```python
from build123d import *

# Parameters (mm, degrees)
F1_DEPTH    = 30
F2_R        = 10
F3_T1_DEPTH = 56.2345635929
F3_T3_DEPTH = 50.7373541457
F3_T5_DEPTH = 44.5080633868
F3_T7_DEPTH = 55
F4_R        = 1


# Not quite as in the source:
# - a fillet or chamfer that OpenCascade refuses, or shapes differently, is made with other operations: its cross-section is extruded or revolved along the edge and cut away or added


with BuildPart() as f1:
    # F0 (on Right) → F1 (new body)
    with BuildSketch(Plane.YZ):
        Polygon((-27.3037352718, 5), (-27.0568225533, 0), (42.9431774467, 0), (42.9431774467, 5), (25.6962647282, 5), (45.6962647282, 40), (40.6962647282, 40), (20.6962647282, 5), (8.8888889937, 5), (2.6962647282, 5), (2.6962647282, 40), (-2.3037352718, 40), (-2.3037352718, 5), align=None)
    extrude(amount=F1_DEPTH)

    # F2
    f2_edges = [f1.edges().sort_by_distance(p)[0] for p in [
        (15, 25.696265, 5),
        (15, -2.303735, 5),
    ]]
    fillet(f2_edges, radius=F2_R)

    # F3: fillet of radius 5 on 4 edges, made by hand

    # F3_s2 → F3_t1 (cut)
    with BuildSketch(Plane.YZ.offset(-13.1172817964)):
        with BuildLine():
            ThreePointArc((-22.0568225533, 5), (-25.5923564592, 3.5355339059), (-27.0568225533, 0))
            Line((-27.0568225533, 0), (-27.3037352718, 5))
            Line((-27.3037352718, 5), (-22.0568225533, 5))
        make_face()
    extrude(amount=F3_T1_DEPTH, mode=Mode.SUBTRACT)

    # F3_s4 → F3_t3 (cut)
    with BuildSketch(Plane.YZ.offset(-10.3686770729)):
        with BuildLine():
            ThreePointArc((42.9431774467, 0.8525291709), (42.0241172961, 3.7414614903), (39.6048054683, 5.5683527806))
            Line((39.6048054683, 5.5683527806), (39.7709682705, 6.0399351415))
            ThreePointArc((39.7709682705, 6.0399351415), (42.9280615114, 5.5), (42.9431774467, 5.5))
            Line((42.9431774467, 5.5), (43.4431774467, 5))
            Line((43.4431774467, 5), (43.4431774467, 0.8525291709))
            Line((43.4431774467, 0.8525291709), (42.9431774467, 0.8525291709))
        make_face()
    extrude(amount=F3_T3_DEPTH, mode=Mode.SUBTRACT)

    # F3_s6 → F3_t5 (cut)
    with BuildSketch(Plane.YZ.offset(-7.2540316934)):
        with BuildLine():
            ThreePointArc((39.2566616949, 37.4806946918), (41.0882433145, 39.3245504656), (43.5978774055, 40))
            Line((43.5978774055, 40), (40.6962647282, 40))
            Line((40.6962647282, 40), (39.2566616949, 37.4806946918))
        make_face()
    extrude(amount=F3_T5_DEPTH, mode=Mode.SUBTRACT)

    # F3_s8 → F3_t7 (cut)
    with BuildSketch(Plane.YZ.offset(-12.5)):
        with BuildLine():
            ThreePointArc((-2.3037352718, 35), (-0.8392691778, 38.5355339059), (2.6962647282, 40))
            Line((2.6962647282, 40), (-2.3037352718, 40))
            Line((-2.3037352718, 40), (-2.3037352718, 35))
        make_face()
    extrude(amount=F3_T7_DEPTH, mode=Mode.SUBTRACT)

    # F4
    f4_edges = [f1.edges().sort_by_distance(p)[0] for p in [
        (15, 2.696265, 5),
        (15, 20.696265, 5),
        (15, 2.696265, 40),
        (15, 45.696265, 40),
    ]]
    fillet(f4_edges, radius=F4_R)


solid = f1.part
```
CAD build for the part. Positions are in the model's coordinates, mm. A direction names the side the tool comes from. Coordinates: 2 decimals unless noted, no trailing zeros. Loops run counter-clockwise (first coordinate to the right, second up) from the corner with the lowest first, then second, coordinate; pieces in that order, holes last. Notation, with made-up numbers: (-0.5, 32) - (51.5, 32) arc R12 cw to (51.5, 36) - close; hole circle Ø9 at (6.5, -20.5). An arc over 180 degrees is marked (long way). Return JSON: item names as keys, results as strings.
1. Mould opens along Y. For faces 4 (the cylindrical face through (14.79, 41.06, 39.31)), 5 (the cylindrical face through (14.79, 42.049, 3.706)), 6 (the flat face through (30, 14, 4)) say: released by +Y, released by -Y, zero draft, split by the parting line, or undercut.
Result:
{"face 4": "undercut", "face 5": "released by +Y", "face 6": "zero draft"}
2. 3-axis set-ups, long thin cutter, end or side, ignore diameter. For faces 1 (the flat face through (14.79, 39.469, 29.103)), 2 (the flat face through (15, -2.304, 25)), 3 (the flat face through (15, 2.696, 22)): which of +Z, -Z, +X, -X, +Y, -Y reach the whole face in a straight line?
Result:
{"face 1": "+X, -X, +Y", "face 2": "+Z, +X, -X, -Y", "face 3": "+Z, +X, -X"}
3. Band-saw the part on D-D (z = 36). Give the cut face in (x, y), and give its area (3 significant figures).
Result:
{"outline": "(0, -2.2) - (30, -2.2) - (30, 2.7) - (0, 2.7) - close; (0, 38.41) - (30, 38.41) - (30, 43.41) - (0, 43.41) - close", "area": "297 mm2"}
4. Band-saw the part on B-B (x = 9.5). Give the cut face in (y, z).
Result:
{"outline": "(-27.06, 0) - (42.94, 0) - (42.94, 0.85) arc R5 ccw to (39.6, 5.57) arc R10 cw to (34.25, 19.96) - (44.84, 38.5) arc R1 ccw to (43.97, 40) - (43.6, 40) arc R5 ccw to (39.26, 37.48) - (20.98, 5.5) arc R1 cw to (20.12, 5) - (3.7, 5) arc R1 cw to (2.7, 6) - (2.7, 38.87) arc R1 ccw to (1.45, 39.84) arc R5 ccw to (-2.3, 35) - (-2.3, 15) arc R10 cw to (-12.3, 5) - (-22.06, 5) arc R5 ccw to start"}
5. Band-saw the part on C-C (y = 10). Give the cut face in (x, z), and give its area (3 significant figures).
Result:
{"outline": "(0, 0) - (30, 0) - (30, 5) - (0, 5) - close", "area": "150 mm2"}
6. Drop flat-ended pins along their axis: pin 1 (8 mm diameter, centred on x = 10.5, y = -15, fed in from +Z); pin 2 (9 mm diameter, centred on x = 19.5, z = 24.5, fed in from +Y); pin 3 (0.7 mm diameter, centred on x = 20, z = 0.5, fed in from +Y). Give the stop position or say it passes through.
Result:
{"pin 1": "stops at z = 5.09", "pin 2": "stops at y = 39.41", "pin 3": "stops at y = 42.94"}
7. Probe L1, parallel to Y at x = 23, z = 32; L2, parallel to Y at x = 9.5, z = 34.5; L3, parallel to Z at x = 27, y = 39.5. List the from-to ranges inside material, lowest first. Write a range as from..to.
Result:
{"L1": "y = -2.3..2.7, 36.12..41.12", "L2": "y = -2.3..2.7, 37.55..42.55", "L3": "z = 0..5.61, 29.16..37.86"}
8. Band-saw the part on A-A (z = 28). Give the cut face in (x, y), and give its area (3 significant figures).
Result:
{"outline": "(0, -2.3) - (30, -2.3) - (30, 2.7) - (0, 2.7) - close; (0, 33.84) - (30, 33.84) - (30, 38.84) - (0, 38.84) - close", "area": "300 mm2"}
